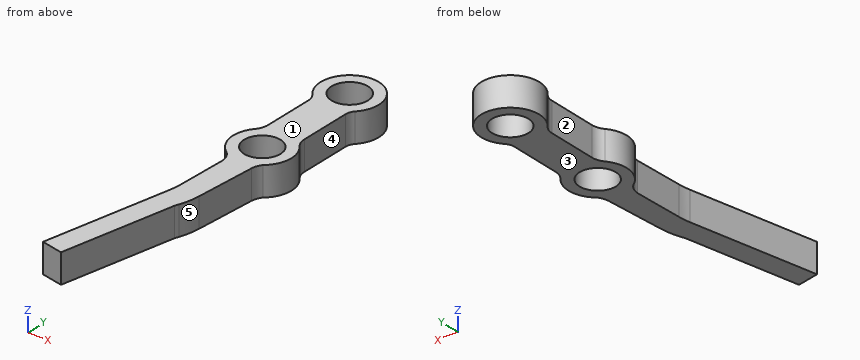
from build123d import *

# Parameters (mm, degrees)
SKETCH_1_R      = 2.5
EXTRUDE_1_DEPTH = 4


with BuildPart() as part:
    # 草图1 → 凸台-拉伸1 (new body)
    with BuildSketch(Plane.XY):
        with BuildLine():
            Line((1.48766526, -12.45557816), (2.043160586, -4.166239224))
            ThreePointArc((2.043160586, -4.166239224), (2.195630301, -3.470719779), (2.545454545, -2.850544554))
            ThreePointArc((2.545454545, -2.850544554), (3.98389954, -0.123518663), (3.05546146, 2.81651483))
            ThreePointArc((3.05546146, 2.81651483), (2.643225677, 3.526362386), (2.5, 4.334637277))
            Line((2.5, 4.334637277), (2.5, 11.411754756))
            ThreePointArc((2.5, 11.411754756), (2.612083111, 12.004318679), (2.932846289, 12.515009985))
            ThreePointArc((2.932846289, 12.515009985), (0.073861123, 19.234330318), (-3.03128037, 12.625158038))
            ThreePointArc((-3.03128037, 12.625158038), (-2.637104468, 11.957199077), (-2.5, 11.19382094))
            Line((-2.5, 11.19382094), (-2.5, 4.337916945))
            ThreePointArc((-2.5, 4.337916945), (-2.643562436, 3.527132911), (-3.056792932, 2.814938078))
            ThreePointArc((-3.056792932, 2.814938078), (-3.974554812, -0.215447508), (-2.401879608, -2.963577121))
            ThreePointArc((-2.401879608, -2.963577121), (-1.721128393, -3.761289924), (-1.445511633, -4.773121596))
            Line((-1.445511633, -4.773121596), (-1.663239971, -11.663933953))
            ThreePointArc((-1.663239971, -11.663933953), (-1.724028802, -12.493204072), (-1.853501284, -13.314557278))
            Line((-1.853501284, -13.314557278), (-5.343304788, -30.714907241))
            Line((-5.343304788, -30.714907241), (-2.401879608, -31.304837669))
            Line((-2.401879608, -31.304837669), (0.728861428, -15.694792688))
            Line((0.728861428, -15.694792688), (0.903082999, -15.217807594))
            ThreePointArc((0.903082999, -15.217807594), (1.293351086, -13.857428153), (1.48766526, -12.45557816))
        make_face()
        with Locations((0, 0.235012309)):
            Circle(SKETCH_1_R, mode=Mode.SUBTRACT)
        with Locations((0, 15.235012309)):
            Circle(SKETCH_1_R, mode=Mode.SUBTRACT)
    extrude(amount=EXTRUDE_1_DEPTH)


solid = part.part
Could you check a few things on this model? Use its own coordinates, in mm. Face numbers are marked on the shaded views. A direction names the side the tool comes from. Give positions to 0.01 mm unless a question says otherwise; leave off trailing zeros. Order: outer loops, then holes, each group sorted by start corner. A loop starts at its lowest first (then second) coordinate and runs counter-clockwise, first axis right, second up.
1. Which directions (+Z, -Z, +X, -X, +Y, -Y) give clear straight access to the entire face, cutting with the end or side of a thin tool? Please do the marked faces 1 and 2.
Answers below:
face 1: +Z, +X, -X, +Y, -Y
face 2: +Z, -Z, -X
2. Suppose I cut it at D-D (y = -19). Write out the boundary of the cut face in (x, z), plus the area to 3 significant figures.
Answers below:
outline: (-2.99, 0) - (0.07, 0) - (0.07, 4) - (-2.99, 4) - close
area: 12.2 mm2
3. Suppose I cut it at B-B (z = 0.9). Write out the boundary of the cut face in (x, y) (1 decimal), plus the area to 3 significant figures.
Answers below:
outline: (-5.3, -30.7) - (-2.4, -31.3) - (0.7, -15.7) - (0.9, -15.2) arc R10 ccw to (1.5, -12.5) - (2, -4.2) arc R2.4 cw to (2.5, -2.9) arc R4 ccw to (3.1, 2.8) arc R2.4 cw to (2.5, 4.3) - (2.5, 11.4) arc R1.6 cw to (2.9, 12.5) arc R4 ccw (long way) to (-3, 12.6) arc R2.2 cw to (-2.5, 11.2) - (-2.5, 4.3) arc R2.4 cw to (-3.1, 2.8) arc R4 ccw to (-2.4, -3) arc R2.4 cw to (-1.4, -4.8) - (-1.7, -11.7) arc R10 cw to (-1.9, -13.3) - close; hole circle Ø5 at (0, 0.2); hole circle Ø5 at (0, 15.2)
area: 187 mm2
4. Suppose I cut it at A-A (x = 0). Write out the boundary of the cut face in (y, z), plus the area to 3 significant figures.
Answers below:
outline: (-19.33, 0) - (-2.26, 0) - (-2.26, 4) - (-19.33, 4) - close; (2.74, 0) - (12.74, 0) - (12.74, 4) - (2.74, 4) - close; (17.74, 0) - (19.24, 0) - (19.24, 4) - (17.74, 4) - close
area: 114 mm2
5. I need wall thicknesses on L1, parallel to X at y = 9, z = 3.85; L2, parallel to Y at x = 3.25, z = 1.85; L3, parallel to Y at x = 2.25, z = 1.2. Which ranges of each line are inside material? Lowest first, please.
Answers below:
L1: x = -2.5 to 2.5
L2: y = -2.1 to 2.57, 12.9 to 17.57
L3: y = -3.34 to -0.85, 1.32 to 14.15, 16.32 to 18.54
6. For pin 1 (1 mm diameter, centred on x = -2.5, y = 12, fed in from -Z); pin 2 (1 mm diameter, centred on x = -3.5, z = 1.5, fed in from +Y); pin 3 (1 mm diameter, centred on y = -5.5, z = 3, fed in from -X); pin 4 (1 mm diameter, centred on y = 7.5, z = 2.5, fed in from -X), each with a flat end and sliding along its axis, tell me the tip position at first contact or that it passes through.
Answers below:
pin 1: stops at z = 0
pin 2: stops at y = 17.88
pin 3: stops at x = -1.48
pin 4: stops at x = -2.5
7. Suppose I cut it at C-C (y = 3.5). Write out the boundary of the cut face in (x, z).
Answers below:
outline: (-2.65, 0) - (2.65, 0) - (2.65, 4) - (-2.65, 4) - close
8. Thinking about a two-plate mould opening in Y: for the marked faces 3, 4 and 5, which applies, +Y half, -Y half, draft (parallel to the pull), parting line (faces both ways), or undercut?
Answers below:
face 3: draft
face 4: undercut
face 5: -Y half
